Geometry: final body of the model. Coordinates: model frame, mm. A direction names the side the tool comes from. Give positions to 0.01 mm unless a question says otherwise; leave off trailing zeros. Write each loop counter-clockwise with the first axis right and the second up, starting at its lowest first coordinate (ties: lowest second). Pieces come first, ordered by that corner, then holes.
```python
from build123d import *

# Parameters (mm, degrees)
SKETCH1_R               = 15
SKETCH1_R_2             = 1.75
SKETCH1_R_3             = 7
BOSS_EXTRUDE1_DEPTH     = 3
SKETCH1_3_R             = 7
SKETCH1_3_R_2           = 3
BOSS_EXTRUDE2_DEPTH     = 13
CUT_EXTRUDE1_DEPTH      = 25.879710609
CUT_EXTRUDE1_DEPTH_BACK = 25.879710609
SKETCH2_R               = 2.25


with BuildPart() as part:
    # Sketch1 → Boss-Extrude1 (new body)
    with BuildSketch(Plane(origin=(0, 0, 0), x_dir=(1, 0, 0), z_dir=(0, 1, 0))):
        with Locations(Location((0, 0, 0), (0, 0, 270))):
            Circle(SKETCH1_R)
        with Locations(Location((-8.660254038, 5, 0), (0, 0, 270))):
            Circle(SKETCH1_R_2, mode=Mode.SUBTRACT)
        with Locations(Location((-8.660254038, -5, 0), (0, 0, 270))):
            Circle(SKETCH1_R_2, mode=Mode.SUBTRACT)
        with Locations(Location((0, -10, 0), (0, 0, 270))):
            Circle(SKETCH1_R_2, mode=Mode.SUBTRACT)
        with Locations(Location((8.660254038, -5, 0), (0, 0, 270))):
            Circle(SKETCH1_R_2, mode=Mode.SUBTRACT)
        with Locations(Location((8.660254038, 5, 0), (0, 0, 270))):
            Circle(SKETCH1_R_2, mode=Mode.SUBTRACT)
        with Locations(Location((0, 10, 0), (0, 0, 270))):
            Circle(SKETCH1_R_2, mode=Mode.SUBTRACT)
        with Locations(Location((0, 0, 0), (0, 0, 270))):
            Circle(SKETCH1_R_3, mode=Mode.SUBTRACT)
    extrude(amount=BOSS_EXTRUDE1_DEPTH)

    # Sketch1_3 → Boss-Extrude2 (add)
    with BuildSketch(Plane(origin=(0, 0, 0), x_dir=(1, 0, 0), z_dir=(0, 1, 0))):
        with Locations(Location((0, 0, 0), (0, 0, 90))):
            Circle(SKETCH1_3_R)
        with Locations(Location((0, 0, 0), (0, 0, 90))):
            Circle(SKETCH1_3_R_2, mode=Mode.SUBTRACT)
    extrude(amount=BOSS_EXTRUDE2_DEPTH)

    # Sketch2 → Cut-Extrude1 (cut, two sides: drawn at the far end of the back side and taken through both)
    with BuildSketch(Plane(origin=(0, 0, 0), x_dir=(0, 0, -1), z_dir=(1, 0, 0)).offset(-CUT_EXTRUDE1_DEPTH_BACK)):
        with Locations((0, 8)):
            Circle(SKETCH2_R)
    extrude(amount=CUT_EXTRUDE1_DEPTH + CUT_EXTRUDE1_DEPTH_BACK, mode=Mode.SUBTRACT)


solid = part.part
```
Item 1: Pull-direction query (X, two-part tool) for faces 3 (the face through (0, 6, 3)), 4 (the face through (2.681, 7.93, -6.466)), 5 (the face through (4.46, 10.23, 0.29)); classes: +X half, -X half, draft (parallel to the pull), parting line (faces both ways), or undercut.
Found:
face 3: undercut
face 4: parting line
face 5: draft
Item 2: Line query: L1, parallel to X at y = 1.8, z = -5; L2, parallel to Z at x = 8.25, y = 0.75; L3, parallel to Y at x = -3.25, z = -12.5. Output: solid intervals per line, ascending.
Found:
L1: x = -14.14 to -10.41, -6.91 to 6.91, 10.41 to 14.14
L2: z = -12.53 to -6.7, -3.3 to 3.3, 6.7 to 12.53
L3: y = 0 to 3
Item 3: Section A-A, the plane x = 0. Return the cut outline in (y, z).
Found:
outline: (0, -15) - (3, -15) - (3, -11.75) - (0, -11.75) - close; (0, -8.25) - (3, -8.25) - (3, -7) - (13, -7) - (13, -3) - (0, -3) - close; (0, 3) - (13, 3) - (13, 7) - (3, 7) - (3, 8.25) - (0, 8.25) - close; (0, 11.75) - (3, 11.75) - (3, 15) - (0, 15) - close
Item 4: Section D-D, the plane x = 9.5. Return the cut outline in (y, z).
Found:
outline: (0, -11.61) - (3, -11.61) - (3, -6.54) - (0, -6.54) - close; (0, -3.46) - (3, -3.46) - (3, 3.46) - (0, 3.46) - close; (0, 6.54) - (3, 6.54) - (3, 11.61) - (0, 11.61) - close
Item 5: Pin query (flat end, axial travel): pin 1 Ø5.5 at (x, z) = (0, -10) entering from -Y; pin 2 Ø6 at (y, z) = (2, -7.5) entering from +X; pin 3 Ø2 at (y, z) = (11, 1) entering from -X; pin 4 Ø5 at (y, z) = (10, 1) entering from +X. Return the tip coordinate at first contact, or that it passes through.
Found:
pin 1: stops at y = 0
pin 2: stops at x = 14.31
pin 3: stops at x = -7
pin 4: stops at x = 7
Item 6: Section B-B, the plane z = 6. Return the cut outline in (x, y).
Found:
outline: (-13.75, 0) - (-10.1, 0) - (-10.1, 3) - (-13.75, 3) - close; (-7.22, 0) - (7.22, 0) - (7.22, 3) - (3.61, 3) - (3.61, 13) - (-3.61, 13) - (-3.61, 3) - (-7.22, 3) - close; (10.1, 0) - (13.75, 0) - (13.75, 3) - (10.1, 3) - close
Item 7: Reachability of faces 1 (the face through (-7.48, 1.48, 3.71)), 2 (the face through (-6.5, 3, 3.1)) from +Z, -Z, +X, -X, +Y, -Y: full face, straight path, thin tool, end or side. Return the list, or none.
Found:
face 1: +Y, -Y
face 2: +Y
Item 8: Section C-C, the plane y = 7.5. Return the cut outline in (x, z).
Found:
outline: (-6.65, -2.19) arc R7 ccw to (6.65, -2.19) - (2.05, -2.19) arc R3 cw to (-2.05, -2.19) - close; (-6.65, 2.19) - (-2.05, 2.19) arc R3 cw to (2.05, 2.19) - (6.65, 2.19) arc R7 ccw to start
